The listing builds one solid part. Answer for the finished solid, in the listing's coordinates (mm). A direction names the side the tool comes from. Give positions to 0.01 mm unless a question says otherwise; leave off trailing zeros. Order: outer loops, then holes, each group sorted by start corner. A loop starts at its lowest first (then second) coordinate and runs counter-clockwise, first axis right, second up. Notation, with made-up numbers: (-26, -4) - (-13, -4) arc R9 cw to (-13, 11) - close; hole circle Ø7 at (89, 18). An arc over 180 degrees is marked (long way). Answer as a JSON object with one key per item and string values. Group by question number.
Q1. The mould has two halves that part along X. Classify faces 6 (the face through (21.994, -11.958, 2.281)), 7 (the face through (36, -2, 36.6)), 8 (the face through (31.84, 7.67, 25.06)): released by +X, released by -X, zero draft, split by the parting line, or undercut.
Q2. Consider line 1 (Z direction, x = -8, y = 2); line 2 (X direction, y = 2, z = 37); line 3 (Y direction, x = 37, z = 19.5). Determine where each line is inside the solid, lowest interval first.
Q3. A cutting plane is placed at C-C, the plane y = -6.5. Give the vertices of the cut face in (x, z).
Q4. A cutting plane is placed at D-D, the plane z = 37.5. Give the vertices of the cut face in (x, y).
Q5. A cutting plane is placed at A-A, the plane x = 44.4. Give the vertices of the cut face in (y, z), and give its area (3 significant figures).
Q6. For faces 1 (the face through (24.4, -9, 11)), 2 (the face through (14.4, -24, 25)), 3 (the face through (37, -1, 32)), 4 (the face through (-1.041, 7.719, 2.406)), 5 (the face through (24.4, -9, 40)), determine the directions among +Z, -Z, +X, -X, +Y, -Y from which every point of the face is accessible in a straight line to the end or side of a thin tool.
Q7. Given pin 1 (5 mm diameter, centred on x = 20.5, z = 41.5, fed in from +Y); pin 2 (6.5 mm diameter, centred on x = 32.5, y = -3.5, fed in from -Z); pin 3 (8.5 mm diameter, centred on x = 33, z = 21.5, fed in from -Y); pin 4 (12 mm diameter, centred on x = 2, y = 2.5, fed in from -Z), each flat-ended and moving along its own axis, determine where each tip first touches the part or whether it passes through.
Q8. A cutting plane is placed at B-B, the plane z = 29. Give the vertices of the cut face in (x, y).
Autodesk Inventor part; units mm, degrees
ref_plane "YZ Plane" through (0, 0, 0) normal (1, 0, 0) x (0, 1, 0)
ref_plane "XZ Plane" through (0, 0, 0) normal (0, 1, 0) x (-1, 0, 0)
ref_plane "XY Plane" through (0, 0, 0) normal (0, 0, 1) x (1, 0, 0)
sketch "Szkic1" plane through (0, 0, 0) normal (0, 0, 1) x (1, 0, 0)
  point P0 (0, 0)
sketch "Szkic2" plane through (0, 0, 0) normal (0, 0, 1) x (1, 0, 0)
  line L0 (-18, 0) -> (0, 0)
  line L1 (0, 0) -> (14.4, -14.4)
  line L2 (14.4, -14.4) -> (14.4, -34.4)
  line L3 (14.4, -34.4) -> (24.4, -34.4)
  line L4 (24.4, -34.4) -> (24.4, 0)
  line L5 (24.4, 0) -> (24.4, 10)
  line L6 (24.4, 10) -> (-18, 10)
  line L7 (-18, 10) -> (-18, 0)
  dimension "d0" = 14.4
  dimension "d1" = 14.4
  dimension "d2" = 18
  dimension "d3" = 20
  dimension "d4" = 10
  dimension "d5" = 10
extrude "Wyciągnięcie proste1" add sketch "Szkic2" along normal blind 51.2
sketch "Szkic3" plane through (24.4, -34.4, 0) normal (1, 0, 0) x (0, 0, -1)
  line L0 (0, 44.4) -> (0, 0)
  line L1 (0, 44.4) -> (-51.2, 44.4)
  line L2 (-51.2, 0) -> (-51.2, 44.4)
  line L3 (0, 0) -> (-51.2, 0)
  line L4 (-36.6, 44.4) -> (-14.6, 44.4)
  line L5 (-14.6, 44.4) -> (-14.6, 22.4)
  line L6 (-14.6, 22.4) -> (-36.6, 22.4)
  line L7 (-36.6, 22.4) -> (-36.6, 44.4)
  point P0 (0, 34.4)
  point P1 (-25.6, 44.4)
  dimension "d8" = 22
  dimension "d9" = 22
extrude "Wyciągnięcie proste2" add sketch "Szkic3" along normal blind 25 contours L5 L6 L7 L1
sketch "Szkic4" plane through (49.4, -34.4, 0) normal (1, 0, 0) x (0, 0, -1)
  line L0 (-14.6, 44.4) -> (-36.6, 44.4)
  line L1 (-36.6, 44.4) -> (-36.6, 22.4)
  line L2 (-36.6, 22.4) -> (-14.6, 22.4)
  line L3 (-14.6, 22.4) -> (-14.6, 44.4)
  line L4 (-32, 39.8) -> (-19.2, 39.8)
  line L5 (-19.2, 39.8) -> (-19.2, 27)
  line L6 (-19.2, 27) -> (-32, 27)
  line L7 (-32, 27) -> (-32, 39.8)
  point P0 (0, 34.4)
  point P1 (-25.6, 39.8)
  point P2 (-25.6, 44.4)
  point P3 (-19.2, 33.4)
  point P4 (-14.6, 33.4)
  dimension "d12" = 12.8
  dimension "d13" = 12.8
extrude "Wyciągnięcie proste3" cut sketch "Szkic4" against normal blind 26 contours L4 L5 L6 L7
sketch "Szkic5" plane through (-18, 10, 0) normal (0, 1, 0) x (1, 0, 0)
  line L0 (0, 0) -> (42.4, 0)
  line L1 (0, 0) -> (0, -51.2)
  line L2 (42.4, -51.2) -> (0, -51.2)
  line L3 (42.4, -36.6) -> (42.4, -51.2)
  line L4 (42.4, -36.6) -> (67.4, -36.6)
  line L5 (67.4, -14.6) -> (67.4, -36.6)
  line L6 (42.4, -14.6) -> (67.4, -14.6)
  line L7 (42.4, 0) -> (42.4, -14.6)
  line L8 (18, 0) -> (18, -51.2)
  point P0 (9.9, -37.2)
  point P1 (9.9459, -23.2)
  dimension "d17" = 8.1
  dimension "d18" = 14
  dimension "d19" = 14
hole "Otwór1" at (-8.1, 10, 37.2) at (-8.0541, 10, 23.2) direction (0, -1, 0) diameter 3 end through all
chamfer "Faza1" distance 15 angle 30 1 edges at (24.4, -34.4, 25.6) measured on face at (24.4, -26.9333, 21.9333)
fillet "Zaokrąglenie1" radius 8 1 edges at (24.4, -12, 25.6)
fillet "Zaokrąglenie2" radius 8 1 edges at (24.4, -4.7, 51.2)
fillet "Zaokrąglenie3" radius 8 1 edges at (24.4, -4.7, 0)
fillet "Zaokrąglenie4" radius 8 7 edges at (-18, 10, 25.6) (22.0569, 10, 48.8569) (24.4, 10, 39.9) (-0.8, 10, 51.2) (22.0569, 10, 2.3431) (24.4, 10, 11.3) (-0.8, 10, 0)
sketch "Szkic6" plane through (49.4, -34.4, 0) normal (1, 0, 0) x (0, 0, -1)
  line L0 (-32, 27) -> (-32, 39.8)
  line L1 (-32, 39.8) -> (-19.2, 39.8)
  line L2 (-19.2, 39.8) -> (-19.2, 27)
  line L3 (-19.2, 27) -> (-32, 27)
  line L4 (-14.6, 44.4) -> (-36.6, 44.4)
  line L5 (-36.6, 44.4) -> (-36.6, 22.4)
  line L6 (-36.6, 22.4) -> (-14.6, 22.4)
  line L7 (-14.6, 22.4) -> (-14.6, 44.4)
  line L8 (-20.5395, 39.8) -> (-13.1078, 39.8)
  line L9 (-13.1078, 39.8) -> (-13.1078, 27)
  line L10 (-13.1078, 27) -> (-20.5395, 27)
  line L11 (-20.5395, 27) -> (-20.5395, 39.8)
  point P0 (0, 34.4)
extrude "Wyciągnięcie proste4" cut sketch "Szkic6" against normal blind 16 contours L11 L1 L2 L3 | L2 L8 L7 L10 | L7 L8 L9 L10
sketch "Szkic7" plane through (49.4, 10, 36.6) normal (0, 1, 0) x (1, 0, 0)
  line L0 (-33, 0) -> (0, 0)
  line L1 (0, 22) -> (0, 0)
  line L2 (-33, 22) -> (0, 22)
  line L3 (-33, 28.6) -> (-33, 22)
  line L4 (-59.4, 28.6) -> (-33, 28.6)
  line L5 (-59.4, -6.6) -> (-59.4, 28.6)
  line L6 (-33, -6.6) -> (-59.4, -6.6)
  line L7 (-33, 0) -> (-33, -6.6)
  circle A0 centre (-57.5, -0.6) radius 1.5
  circle A1 centre (-57.4541, 13.4) radius 1.5
  point P0 (-49.4, 36.6)
  point P1 (-5, 11)
  point P2 (-20, 11)
  dimension "d36" = 5
  dimension "d37" = 15
hole "Otwór2" at (44.4, 10, 25.6) at (29.4, 10, 25.6) direction (0, -1, 0) diameter 5 depth 8 tip angle 118
properties part number "mocowanie_do_ramy"
Reply:
{
 "1": {"face 6": "released by +X", "face 7": "zero draft", "face 8": "undercut"},
 "2": {"line 1": "z = 0 to 21.7, 24.7 to 35.7, 38.7 to 51.2", "line 2": "x = -18 to -9.59, -6.61 to 24.4", "line 3": "y = -12 to -7.4, 5.4 to 10"},
 "3": {"outline": "(6.5, 0) - (16.4, 0) arc R8 ccw to (24.4, 8) - (24.4, 14.6) - (33.4, 14.6) - (33.4, 19.2) - (23.4, 19.2) - (23.4, 32) - (49.4, 32) - (49.4, 36.6) - (24.4, 36.6) - (24.4, 43.2) arc R8 ccw to (16.4, 51.2) - (6.5, 51.2) - close"},
 "4": {"outline": "(-18, 0) - (-9.57, 0) - (-9.57, 10) - (-10, 10) arc R8 ccw to (-18, 2) - close; (-6.63, 0) - (0, 0) - (14.4, -14.4) - (14.4, -34.4) - (15.74, -34.4) - (24.4, -19.4) - (24.4, 2) arc R8 ccw to (16.4, 10) - (-6.63, 10) - close"},
 "5": {"outline": "(-12, 14.6) - (-7.4, 14.6) - (-7.4, 32) - (5.4, 32) - (5.4, 28.1) - (10, 28.1) - (10, 36.6) - (-12, 36.6) - close; (5.4, 14.6) - (10, 14.6) - (10, 23.1) - (5.4, 23.1) - close", "area": "238 mm^2"},
 "6": {"face 1": "-Z, +X, +Y, -Y", "face 2": "+Z, -Z, -X, -Y", "face 3": "+X", "face 4": "-Z, +X, -X, +Y", "face 5": "+Z, +X, +Y, -Y"},
 "7": {"pin 1": "stops at y = 9.84", "pin 2": "stops at z = 14.6", "pin 3": "stops at y = -12.87", "pin 4": "stops at z = 0"},
 "8": {"outline": "(-18, 0) - (0, 0) - (14.4, -14.4) - (14.4, -34.4) - (15.74, -34.4) - (24.4, -19.4) arc R8 cw to (32.38, -12) - (49.4, -12) - (49.4, -7.4) - (23.4, -7.4) - (23.4, 5.4) - (49.4, 5.4) - (49.4, 10) - (-10, 10) arc R8 ccw to (-18, 2) - close"}
}
